The listing builds one solid part. Answer for the finished solid, in the listing's coordinates (mm). A direction names the side the tool comes from. Coordinates: 2 decimals unless noted, no trailing zeros. Return JSON: item names as keys, results as strings. Group by question number.
1. Find the intervals of material crossed by line 1 along X through (y, z) = (4, 0.6); line 2 along X through (y, z) = (145, 1.45); line 3 along Y through (x, z) = (143, 1.7), in increasing order.
2. Section A-A (z = 0.7) is taken. State how many separate pieces and enclosed holes the cut face has, and give its area (3 significant figures).
3. Each of these flat-tipped pins is pushed along its axis until it touches: P1, Ø3.5, axis at x = 32, y = 50, coming from the -Z side; P2, Ø1.5, axis at y = 34.5, z = 1.5, coming from the +X side; P3, Ø0.9, axis at y = 54, z = 1.5, coming from the -X side; P4, Ø1.5, axis at x = 15, z = 1, coming from the +Y side (3 decimals). Where does it stop, or does it pass through?
4. Which of the six approach directions +Z, -Z, +X, -X, +Y, -Y give full straight-line access (tool end or side, diameter ignored) to faces 4 (the face through (166.5, 23.93, 1.48)), 5 (the face through (40.12, 166.41, 1.48)), 6 (the face through (6.163, 100.642, 1.479)), 7 (the face through (162.255, -14.895, 1.479))?
5. The mould has two halves that part along X. Classify faces 1 (the face through (94, 75, 0)), 2 (the face through (50, -10, 1)), 3 (the face through (166.43, 96, 1.48)): pulls with the +X half, pulls with the -X half, needs draft (parallel to the pull), parting line crosses it, or undercut.
```python
from build123d import *

# Parameters (mm, degrees)
MODEL_R             = 1.5
MODEL_R_2           = 14.5
MODEL_W             = 3
MODEL_H             = 27
MODEL_W_2           = 27
MODEL_H_2           = 3
MODEL_W_3           = 7
MODEL_H_3           = 15
MODEL_W_4           = 19.975
MODEL_H_4           = 6.25
BOSS_EXTRUDE1_DEPTH = 3


with BuildPart() as part:
    # Model → Boss-Extrude1 (new body)
    with BuildSketch(Plane.XY):
        with BuildLine():
            Line((190, 103.697579254), (190, 147.5))
            Line((190, 147.5), (165, 170))
            Line((165, 170), (154.89207995, 162.725031973))
            Line((154.89207995, 162.725031973), (145, 170))
            Line((145, 170), (45, 170))
            Line((45, 170), (35.10792005, 162.725031973))
            Line((35.10792005, 162.725031973), (25, 170))
            Line((25, 170), (0, 147.5))
            Line((0, 147.5), (0, 103.697579254))
            Line((0, 103.697579254), (12.5, 97.5))
            Line((12.5, 97.5), (20, 97.5))
            ThreePointArc((20, 97.5), (23.535533906, 96.035533906), (25, 92.5))
            Line((25, 92.5), (25, 27.5))
            ThreePointArc((25, 27.5), (23.535533906, 23.964466094), (20, 22.5))
            Line((20, 22.5), (12.5, 22.5))
            Line((12.5, 22.5), (0, 17.867533831))
            Line((0, 17.867533831), (0, 0))
            Line((0, 0), (0, -19.5))
            Line((0, -19.5), (3, -22.5))
            Line((3, -22.5), (10, -22.5))
            Line((10, -22.5), (45, -7.5))
            Line((45, -7.5), (55, -12.5))
            Line((55, -12.5), (72.142857143, -12.5))
            Line((72.142857143, -12.5), (90, 0))
            Line((90, 0), (100, 0))
            Line((100, 0), (117.857142857, -12.5))
            Line((117.857142857, -12.5), (135, -12.5))
            Line((135, -12.5), (145, -7.5))
            Line((145, -7.5), (180, -22.5))
            Line((180, -22.5), (187, -22.5))
            Line((187, -22.5), (190, -19.5))
            Line((190, -19.5), (190, 0))
            Line((190, 0), (190, 17.867533831))
            Line((190, 17.867533831), (177.5, 22.5))
            Line((177.5, 22.5), (170, 22.5))
            ThreePointArc((170, 22.5), (166.464466094, 23.964466094), (165, 27.5))
            Line((165, 27.5), (165, 92.5))
            ThreePointArc((165, 92.5), (166.464466094, 96.035533906), (170, 97.5))
            Line((170, 97.5), (177.5, 97.5))
            Line((177.5, 97.5), (190, 103.697579254))
        make_face()
        with Locations((32, 50)):
            Circle(MODEL_R, mode=Mode.SUBTRACT)
        with Locations((47, 50)):
            Circle(MODEL_R, mode=Mode.SUBTRACT)
        with Locations((32, 70)):
            Circle(MODEL_R, mode=Mode.SUBTRACT)
        with Locations((47, 70)):
            Circle(MODEL_R, mode=Mode.SUBTRACT)
        with Locations((158, 70)):
            Circle(MODEL_R, mode=Mode.SUBTRACT)
        with Locations((143, 70)):
            Circle(MODEL_R, mode=Mode.SUBTRACT)
        with Locations((158, 50)):
            Circle(MODEL_R, mode=Mode.SUBTRACT)
        with Locations((143, 50)):
            Circle(MODEL_R, mode=Mode.SUBTRACT)
        with Locations((45, 140)):
            Circle(MODEL_R_2, mode=Mode.SUBTRACT)
        with Locations((31.211417767, 126.211417767)):
            Circle(MODEL_R, mode=Mode.SUBTRACT)
        with Locations((58.788582233, 153.788582233)):
            Circle(MODEL_R, mode=Mode.SUBTRACT)
        with Locations((145, 140)):
            Circle(MODEL_R_2, mode=Mode.SUBTRACT)
        with Locations((158.788582233, 126.211417767)):
            Circle(MODEL_R, mode=Mode.SUBTRACT)
        with Locations((131.211417767, 153.788582233)):
            Circle(MODEL_R, mode=Mode.SUBTRACT)
        with Locations((65.995999264, 37.286813453)):
            Circle(MODEL_R, mode=Mode.SUBTRACT)
        with Locations((65.995999264, 19.661813453)):
            Circle(MODEL_R, mode=Mode.SUBTRACT)
        with Locations((121.395999264, 37.386813453)):
            Circle(MODEL_R, mode=Mode.SUBTRACT)
        with Locations((121.595999264, 19.661813453)):
            Circle(MODEL_R, mode=Mode.SUBTRACT)
        with Locations((65.995999264, 85.107027522)):
            Circle(MODEL_R, mode=Mode.SUBTRACT)
        with Locations((65.995999264, 102.732027522)):
            Circle(MODEL_R, mode=Mode.SUBTRACT)
        with Locations((121.395999264, 102.832027522)):
            Circle(MODEL_R, mode=Mode.SUBTRACT)
        with Locations((121.595999264, 85.107027522)):
            Circle(MODEL_R, mode=Mode.SUBTRACT)
        with Locations((4.5, 126.5)):
            Rectangle(MODEL_W, MODEL_H, mode=Mode.SUBTRACT)
        with Locations((185.5, 126.5)):
            Rectangle(MODEL_W, MODEL_H, mode=Mode.SUBTRACT)
        with Locations((95, 165.5)):
            Rectangle(MODEL_W_2, MODEL_H_2, mode=Mode.SUBTRACT)
        with Locations((76.6, 99.390878679)):
            Rectangle(MODEL_W_3, MODEL_H_3, mode=Mode.SUBTRACT)
        with Locations((85.8, 99.390878679)):
            Rectangle(MODEL_W_3, MODEL_H_3, mode=Mode.SUBTRACT)
        with Locations((95, 99.390878679)):
            Rectangle(MODEL_W_3, MODEL_H_3, mode=Mode.SUBTRACT)
        with Locations((104.2, 99.390878679)):
            Rectangle(MODEL_W_3, MODEL_H_3, mode=Mode.SUBTRACT)
        with Locations((113.4, 99.390878679)):
            Rectangle(MODEL_W_3, MODEL_H_3, mode=Mode.SUBTRACT)
        with Locations((95.108499264, 86.757027522)):
            Rectangle(MODEL_W_4, MODEL_H_4, mode=Mode.SUBTRACT)
        with Locations((76.6, 33.94566461)):
            Rectangle(MODEL_W_3, MODEL_H_3, mode=Mode.SUBTRACT)
        with Locations((85.8, 33.94566461)):
            Rectangle(MODEL_W_3, MODEL_H_3, mode=Mode.SUBTRACT)
        with Locations((95, 33.94566461)):
            Rectangle(MODEL_W_3, MODEL_H_3, mode=Mode.SUBTRACT)
        with Locations((104.2, 33.94566461)):
            Rectangle(MODEL_W_3, MODEL_H_3, mode=Mode.SUBTRACT)
        with Locations((113.4, 33.94566461)):
            Rectangle(MODEL_W_3, MODEL_H_3, mode=Mode.SUBTRACT)
        with Locations((95.108499264, 21.311813453)):
            Rectangle(MODEL_W_4, MODEL_H_4, mode=Mode.SUBTRACT)
        with BuildLine():
            Line((80, 119.172827764), (80, 135.172827764))
            ThreePointArc((80, 135.172827764), (80.585786438, 136.587041326), (82, 137.172827764))
            Line((82, 137.172827764), (108, 137.172827764))
            ThreePointArc((108, 137.172827764), (109.414213562, 136.587041326), (110, 135.172827764))
            Line((110, 135.172827764), (110, 119.172827764))
            ThreePointArc((110, 119.172827764), (109.414213562, 117.758614202), (108, 117.172827764))
            Line((108, 117.172827764), (82, 117.172827764))
            ThreePointArc((82, 117.172827764), (80.585786438, 117.758614202), (80, 119.172827764))
        make_face(mode=Mode.SUBTRACT)
        with Locations((4.5, 1.875)):
            Rectangle(MODEL_W, MODEL_H, mode=Mode.SUBTRACT)
        with Locations((185.5, 1.875)):
            Rectangle(MODEL_W, MODEL_H, mode=Mode.SUBTRACT)
    extrude(amount=BOSS_EXTRUDE1_DEPTH)


solid = part.part
```
The answers:
{
 "1": {"line 1": "x = 0 to 3, 6 to 184, 187 to 190", "line 2": "x = 0 to 31.39, 58.61 to 131.39, 158.61 to 190", "line 3": "y = -8.5 to 48.5, 51.5 to 68.5, 71.5 to 125.64, 154.36 to 170"},
 "2": {"separate pieces": "1", "enclosed holes": "40", "area": "26,300 mm2"},
 "3": {"P1": "stops at z = 0", "P2": "stops at x = 165", "P3": "stops at x = 25", "P4": "stops at y = 161.675"},
 "4": {"face 4": "+Z, -Z, +X", "face 5": "+Z, -Z, +Y", "face 6": "+Z, -Z, -X", "face 7": "+Z, -Z, -Y"},
 "5": {"face 1": "needs draft", "face 2": "undercut", "face 3": "pulls with the +X half"}
}
